Design review of the part built by this model. Coordinates are the model's own, in mm. Give positions to 0.01 mm unless a question says otherwise; leave off trailing zeros. Write each loop counter-clockwise with the first axis right and the second up, starting at its lowest first coordinate (ties: lowest second). Pieces come first, ordered by that corner, then holes. Notation, with made-up numbers: (71, -34) - (96, -34) arc R17 cw to (96, -4) - close; hole circle Ø5 at (-27, 39.25). An arc over 180 degrees is marked (long way). Use a Markdown table: item, result. Add a question column.
```python
from build123d import *

# Parameters (mm, degrees)
EXTRUSION1_DEPTH         = 1.6
ESQUISSE3_R              = 2.4
ENL_V_MAT_EXTRU_2_DEPTH  = 3
ESQUISSE4_R              = 2.25
ENL_V_MAT_EXTRU_3_DEPTH  = 10
ENL_V_MAT_EXTRU_4_DEPTH  = 10
ESQUISSE6_R              = 1.55
ENL_V_MAT_EXTRU_5_DEPTH  = 2
ESQUISSE7_R              = 1.8
ENL_V_MAT_EXTRU_6_DEPTH  = 2
ESQUISSE8_W              = 3.6
ESQUISSE8_H              = 12
EXTRUSION2_DEPTH         = 4.5
ESQUISSE10_R             = 4.5
ENL_V_MAT_EXTRU_7_DEPTH  = 0.1
ESQUISSE19_W             = 10.8
ESQUISSE19_H             = 22.7
EXTRUSION12_DEPTH        = 13.2
ESQUISSE23_W             = 8.032982088
ESQUISSE23_H             = 0.2
ENL_V_MAT_EXTRU_10_DEPTH = 0.1
ESQUISSE26_R             = 3.5
ENL_V_MAT_EXTRU_11_DEPTH = 0.1
ENL_V_START              = -0.1
ESQUISSE27_R             = 3.5
ENL_V_MAT_EXTRU_12_DEPTH = 0.1
ESQUISSE30_R             = 0.8
EXTRUSION14_DEPTH        = 1
ESQUISSE32_W             = 13.032086964
ESQUISSE32_H             = 29.119345892
ENL_V_MAT_EXTRU_15_DEPTH = 10
ESQUISSE38_W             = 3.5
ESQUISSE38_H             = 9
EXTRUSION20_DEPTH        = 5
ESQUISSE40_R             = 1.25
ESQUISSE40_W             = 2
ESQUISSE40_H             = 8.965480912
ENL_V_MAT_EXTRU_16_DEPTH = 10
ENL_V_MAT_EXTRU_17_DEPTH = 10


with BuildPart() as part:
    # Esquisse1 → Extrusion1 (new body)
    with BuildSketch(Plane.XY):
        Polygon((45.902468776, -16.999888115), (45.902468776, -184.415394951), (16.22088018, -184.415394951), (16.22088018, -229.296420917), (-51.512423031, -229.296420917), (-51.512423031, -47.949999998), (-63.097644562, -47.949999998), (-63.097644562, -13.499999747), (-80.044329504, -13.499999747), (-80.044329504, 1.914815016), (-47.830041474, 1.914815016), (-47.830041474, -4.796422374), (32.16998758, -4.796422374), (32.16998758, -16.999888115), align=None)
    extrude(amount=EXTRUSION1_DEPTH)

    # Esquisse3 → Enl_v. mat.-Extru.2 (cut)
    with BuildSketch(Plane(origin=(0, 0, 0), x_dir=(-1, 0, 0), z_dir=(0, 0, -1))):
        with Locations((-21.656316362, -141.741425249)):
            Circle(ESQUISSE3_R)
        with Locations((35.493683638, -141.741425249)):
            Circle(ESQUISSE3_R)
        with Locations((-21.656316362, -33.791425249)):
            Circle(ESQUISSE3_R)
        with Locations((35.493683638, -33.791425249)):
            Circle(ESQUISSE3_R)
    extrude(amount=-ENL_V_MAT_EXTRU_2_DEPTH, mode=Mode.SUBTRACT)

    # Esquisse4 → Enl_v. mat.-Extru.3 (cut)
    with BuildSketch(Plane.XY.offset(1.6)):
        with Locations((26.170115332, -26.99975322)):
            Circle(ESQUISSE4_R)
        with Locations((-39.829884666, -27.000195468)):
            Circle(ESQUISSE4_R)
        with Locations((26.171127143, -177.999753216)):
            Circle(ESQUISSE4_R)
        with Locations((-39.828705337, -203.000195464)):
            Circle(ESQUISSE4_R)
    extrude(amount=-ENL_V_MAT_EXTRU_3_DEPTH, mode=Mode.SUBTRACT)

    # Esquisse5 → Enl_v. mat.-Extru.4 (cut)
    with BuildSketch(Plane(origin=(0, 0, 0), x_dir=(-1, 0, 0), z_dir=(0, 0, -1))):
        with BuildLine():
            Line((-8.188160733, -186.837695498), (-8.188160733, -151.837794325))
            ThreePointArc((-8.188160733, -151.837794325), (-6.723694639, -148.30226042), (-3.188160733, -146.837794325))
            Line((-3.188160733, -146.837794325), (30.738384276, -146.837794325))
            ThreePointArc((30.738384276, -146.837794325), (34.273918182, -148.30226042), (35.738384276, -151.837794325))
            Line((35.738384276, -151.837794325), (35.738384276, -186.837695498))
            ThreePointArc((35.738384276, -186.837695498), (34.273918182, -190.373229404), (30.738384276, -191.837695498))
            Line((30.738384276, -191.837695498), (-3.188160733, -191.837695498))
            ThreePointArc((-3.188160733, -191.837695498), (-6.723694639, -190.373229404), (-8.188160733, -186.837695498))
        make_face()
    extrude(amount=-ENL_V_MAT_EXTRU_4_DEPTH, mode=Mode.SUBTRACT)

    # Esquisse6 → Enl_v. mat.-Extru.5 (cut)
    with BuildSketch(Plane.XY.offset(1.6)):
        with Locations((23.399949199, -7.999901551)):
            Circle(ESQUISSE6_R)
        with Locations((-21.600050801, -7.999953529)):
            Circle(ESQUISSE6_R)
    extrude(amount=-ENL_V_MAT_EXTRU_5_DEPTH, mode=Mode.SUBTRACT)

    # Esquisse7 → Enl_v. mat.-Extru.6 (cut)
    with BuildSketch(Plane.XY.offset(1.6)):
        with Locations((-5.456e-06, -10.999928579)):
            Circle(ESQUISSE7_R)
    extrude(amount=-ENL_V_MAT_EXTRU_6_DEPTH, mode=Mode.SUBTRACT)

    # Esquisse8 → Extrusion2 (add)
    with BuildSketch(Plane(origin=(0, 0, 0), x_dir=(-1, 0, 0), z_dir=(0, 0, -1))):
        with Locations((-42.352506676, -152.415391345)):
            Rectangle(ESQUISSE8_W, ESQUISSE8_H)
    extrude(amount=EXTRUSION2_DEPTH)

    # Esquisse10 → Enl_v. mat.-Extru.7 (cut)
    with BuildSketch(Plane.XY.offset(1.6)):
        with Locations((26.169971141, -26.999898346)):
            Circle(ESQUISSE10_R)
        with Locations((-39.830028858, -26.999974585)):
            Circle(ESQUISSE10_R)
        with Locations((26.170145567, -177.999898346)):
            Circle(ESQUISSE10_R)
        with Locations((-39.829825555, -202.999974585)):
            Circle(ESQUISSE10_R)
    extrude(amount=-ENL_V_MAT_EXTRU_7_DEPTH, mode=Mode.SUBTRACT)

    # Esquisse19 → Extrusion12 (add)
    with BuildSketch(Plane(origin=(0, 0, 0), x_dir=(-1, 0, 0), z_dir=(0, 0, -1))):
        with Locations((50.547644562, -34.684676228)):
            Rectangle(ESQUISSE19_W, ESQUISSE19_H)
    extrude(amount=EXTRUSION12_DEPTH)

    # Esquisse23 → Enl_v. mat.-Extru.10 (cut)
    with BuildSketch(Plane.XY.offset(1.6)):
        with Locations((12.204651777, -184.515396319)):
            Rectangle(ESQUISSE23_W, ESQUISSE23_H)
    extrude(amount=-ENL_V_MAT_EXTRU_10_DEPTH, mode=Mode.SUBTRACT)

    # Esquisse26 → Enl_v. mat.-Extru.11 (cut)
    with BuildSketch(Plane(origin=(0, 0, 0), x_dir=(-1, 0, 0), z_dir=(0, 0, -1))):
        with Locations((-26.171127143, -177.999753216)):
            Circle(ESQUISSE26_R)
        with Locations((-21.656316362, -141.741425249)):
            Circle(ESQUISSE26_R)
        with Locations((35.493683638, -141.741425249)):
            Circle(ESQUISSE26_R)
        with Locations((-26.170115332, -26.99975322)):
            Circle(ESQUISSE26_R)
        with Locations((-21.656316362, -33.791425249)):
            Circle(ESQUISSE26_R)
        with Locations((35.493683638, -33.791425249)):
            Circle(ESQUISSE26_R)
        with Locations((39.829884666, -27.000195468)):
            Circle(ESQUISSE26_R)
    extrude(amount=-ENL_V_MAT_EXTRU_11_DEPTH, mode=Mode.SUBTRACT)

    # Esquisse27 → Enl_v. mat.-Extru.12 (cut)
    with BuildSketch(Plane.XY.offset(1.6).offset(ENL_V_START)):
        with Locations(Location((-35.493683638, -33.791425249, 0), (0, 0, 180))):
            Circle(ESQUISSE27_R)
        with Locations(Location((21.656316362, -33.791425249, 0), (0, 0, 180))):
            Circle(ESQUISSE27_R)
        with Locations(Location((-35.493683638, -141.741425249, 0), (0, 0, 180))):
            Circle(ESQUISSE27_R)
        with Locations(Location((21.656316362, -141.741425249, 0), (0, 0, 180))):
            Circle(ESQUISSE27_R)
    extrude(amount=ENL_V_MAT_EXTRU_12_DEPTH, mode=Mode.SUBTRACT)

    # Esquisse30 → Extrusion14 (add)
    with BuildSketch(Plane(origin=(0, 0, 0), x_dir=(-1, 0, 0), z_dir=(0, 0, -1))):
        with Locations(Location((-41.152518707, -181.415394951, 0), (0, 0, 180))):
            Circle(ESQUISSE30_R)
    extrude(amount=EXTRUSION14_DEPTH)

    # Esquisse32 → Enl_v. mat.-Extru.15 (cut)
    with BuildSketch(Plane(origin=(0, 0, 0), x_dir=(-1, 0, 0), z_dir=(0, 0, -1))):
        with Locations((-16.736923724, -217.856098053)):
            Rectangle(ESQUISSE32_W, ESQUISSE32_H)
    extrude(amount=-ENL_V_MAT_EXTRU_15_DEPTH, mode=Mode.SUBTRACT)

    # Esquisse38 → Extrusion20 (add)
    with BuildSketch(Plane(origin=(0, 0, 0), x_dir=(-1, 0, 0), z_dir=(0, 0, -1))):
        with Locations((48.080624066, -77.449999998)):
            Rectangle(ESQUISSE38_W, ESQUISSE38_H)
    extrude(amount=EXTRUSION20_DEPTH)

    # Esquisse40 → Enl_v. mat.-Extru.16 (cut)
    with BuildSketch(Plane(origin=(0, 0, 0), x_dir=(-1, 0, 0), z_dir=(0, 0, -1))):
        with Locations((-30.652432705, -50.799882548)):
            Circle(ESQUISSE40_R)
        with Locations((-26.652432705, -50.799882548)):
            Circle(ESQUISSE40_R)
        with Locations((3.347567295, -50.799882548)):
            Circle(ESQUISSE40_R)
        with Locations((7.347567295, -55.799882548)):
            Circle(ESQUISSE40_R)
        with Locations((-30.652432705, -91.799882548)):
            Circle(ESQUISSE40_R)
        with Locations((-26.652432705, -91.799882548)):
            Circle(ESQUISSE40_R)
        with Locations((3.347567295, -91.799882548)):
            Circle(ESQUISSE40_R)
        with Locations((7.347567295, -86.799882548)):
            Circle(ESQUISSE40_R)
        with Locations((-14.652432705, -86.751416152)):
            Rectangle(ESQUISSE40_W, ESQUISSE40_H)
    extrude(amount=-ENL_V_MAT_EXTRU_16_DEPTH, mode=Mode.SUBTRACT)

    # Esquisse43 → Enl_v. mat.-Extru.17 (cut)
    with BuildSketch(Plane(origin=(0, 0, 0), x_dir=(-1, 0, 0), z_dir=(0, 0, -1))):
        Polygon((56.847644247, -52.137617645), (56.847644247, -32.949999998), (73.023827772, -32.949999998), (73.023826653, -52.137618589), align=None)
    extrude(amount=-ENL_V_MAT_EXTRU_17_DEPTH, mode=Mode.SUBTRACT)


solid = part.part
```
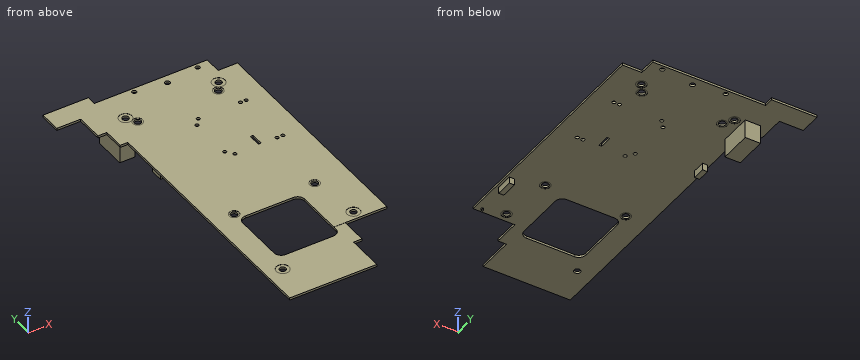
(1) Add section A-A (x = -13). State the section outline as (y, z) points.
(2) For line 1 along Y through (x, z) = (-26, 1); line 2 along Z through (x, y) = (-17, -73); line 3 along Y through (x, z) = (-47.5, -9.25), list the stretches that pass through material, from the lowest coordinate up.
(3) Add section C-C (y = -111). State the section outline as (x, z) points, and give its area (3 significant figures).
(4) Insertion check: pin 1 (0.5 mm diameter, centred on x = 23.5, z = 0.5, fed in from -Y); pin 2 (0.8 mm diameter, centred on y = -1, z = 1, fed in from +X); pin 3 (1.8 mm diameter, centred on y = -214, z = 1, fed in from +X). Each pin has a flat end and moves straight along its axis. Give the tip position at first contact, or say it passes through.
(5) Add section B-B (z = -8.5). State the section outline as (x, y) points.
Answers follow:
| question | item | result |
|---|---|---|
| 1 | outline | (-229.3, 0) - (-191.84, 0) - (-191.84, 1.6) - (-229.3, 1.6) - close; (-146.84, 0) - (-4.8, 0) - (-4.8, 1.6) - (-146.84, 1.6) - close |
| 2 | line 1 | -229.3 to -191.84, -146.84 to -4.8 |
| 2 | line 2 | 0 to 1.6 |
| 2 | line 3 | -46.03 to -23.33 |
| 3 | outline | (-51.51, 0) - (45.9, 0) - (45.9, 1.6) - (-51.51, 1.6) - close |
| 3 | area | 156 mm^2 |
| 4 | pin 1 | y = -184.42 |
| 4 | pin 2 | x = -47.83 |
| 4 | pin 3 | x = 10.22 |
| 5 | outline | (-55.95, -46.03) - (-45.15, -46.03) - (-45.15, -23.33) - (-55.95, -23.33) - close |
